Build history of the part. All positions in model axes, mm. A direction names the side the tool comes from. Coordinates: 2 decimals unless noted, no trailing zeros. Loops run counter-clockwise (first coordinate to the right, second up) from the corner with the lowest first, then second, coordinate; pieces in that order, holes last.
Item 1: Mould opens along Z. For faces 1 (the face through (12.524, 0.986, -39.192)), 2 (the face through (-27.62, 1.01, 53.6)), 3 (the face through (-13.3, 2, 15.6)) say: released by +Z, released by -Z, zero draft, split by the parting line, or undercut.
Item 2: Drill centre lines: line 1 along X through (y, z) = (0.85, 50); line 2 along Z through (x, y) = (2.5, 0.3); line 3 along Z through (x, y) = (10, 0.25). Where is each one in solid material? Low to high.
Item 3: Cut at A-A (x = -6). List the corners of the cut face in (y, z), and give its area (3 significant figures).
Item 4: Cut at C-C (z = 33). List the corners of the cut face in (x, y), and give its area (3 significant figures).
Item 5: Cut at D-D (y = 0.6). Count the separate pieces of the cut face and the enclosed holes in it, and give its area (3 significant figures).
Item 6: 3-axis set-ups, long thin cutter, end or side, ignore diameter. For faces 4 (the face through (29.05, 1, 6)), 5 (the face through (-10.781, -0.507, -8.774)), 6 (the face through (-12.5, 0.99, -15.54)): which of +Z, -Z, +X, -X, +Y, -Y reach the whole face in a straight line?
Item 7: Cut at B-B (z = -27.9). List the corners of the cut face in (x, y).
from build123d import *
from build123d.topology import SkipClean

# Parameters (mm, degrees)
SKETCH3_W           = 58.1
SKETCH3_H           = 99.8
SKETCH3_R           = 1.1
SKETCH3_R_2         = 0.95
SKETCH3_R_3         = 1.4
BOSS_EXTRUDE1_DEPTH = 2
FILLET1_R           = 5
FILLET2_R           = 3
FILLET3_R           = 10
BOSS_EXTRUDE2_START = 1
SKETCH4_R           = 1.6
SKETCH4_R_2         = 0.95
BOSS_EXTRUDE2_DEPTH = 1


with BuildPart() as part:
    # Sketch3 → Boss-Extrude1 (new body)
    with BuildSketch(Plane(origin=(0, 0, 0), x_dir=(1, 0, 0), z_dir=(0, 1, 0))):
        with Locations((0, -5.2)):
            Rectangle(SKETCH3_W, SKETCH3_H)
        with Locations(Location((24.05, -50.1, 0), (0, 0, 270))):
            Circle(SKETCH3_R, mode=Mode.SUBTRACT)
        with Locations(Location((-10.3, -10.3, 0), (0, 0, 270))):
            Circle(SKETCH3_R_2, mode=Mode.SUBTRACT)
        with Locations(Location((13.5, 39.7, 0), (0, 0, 270))):
            Circle(SKETCH3_R, mode=Mode.SUBTRACT)
        with Locations(Location((-13.5, 39.7, 0), (0, 0, 270))):
            Circle(SKETCH3_R, mode=Mode.SUBTRACT)
        with Locations(Location((-24.05, -50.1, 0), (0, 0, 270))):
            Circle(SKETCH3_R, mode=Mode.SUBTRACT)
        with Locations(Location((-24.5, 27.9, 0), (0, 0, 270))):
            Circle(SKETCH3_R_3, mode=Mode.SUBTRACT)
        with Locations(Location((24.5, 27.9, 0), (0, 0, 270))):
            Circle(SKETCH3_R_3, mode=Mode.SUBTRACT)
        with Locations(Location((10.3, 10.3, 0), (0, 0, 270))):
            Circle(SKETCH3_R_2, mode=Mode.SUBTRACT)
        with Locations(Location((10.3, -10.3, 0), (0, 0, 270))):
            Circle(SKETCH3_R_2, mode=Mode.SUBTRACT)
        with Locations(Location((-10.3, 10.3, 0), (0, 0, 270))):
            Circle(SKETCH3_R_2, mode=Mode.SUBTRACT)
        with Locations(Location((-24.5, -30.1, 0), (0, 0, 270))):
            Circle(SKETCH3_R_3, mode=Mode.SUBTRACT)
        with Locations(Location((24.5, -30.1, 0), (0, 0, 270))):
            Circle(SKETCH3_R_3, mode=Mode.SUBTRACT)
        with BuildLine():
            Line((19.05, -45.1), (19.05, -22.090559159))
            Line((19.05, -22.090559159), (8.77972042, -11.82027958))
            ThreePointArc((8.77972042, -11.82027958), (8.77972042, -8.77972042), (11.82027958, -8.77972042))
            Line((11.82027958, -8.77972042), (19.05, -16.009440841))
            Line((19.05, -16.009440841), (19.05, 16.009440841))
            Line((19.05, 16.009440841), (11.82027958, 8.77972042))
            ThreePointArc((11.82027958, 8.77972042), (8.77972042, 8.77972042), (8.77972042, 11.82027958))
            Line((8.77972042, 11.82027958), (19.05, 22.090559159))
            Line((19.05, 22.090559159), (19.05, 34.7))
            Line((19.05, 34.7), (-19.05, 34.7))
            Line((-19.05, 34.7), (-19.05, 22.090559159))
            Line((-19.05, 22.090559159), (-8.77972042, 11.82027958))
            ThreePointArc((-8.77972042, 11.82027958), (-8.77972042, 8.77972042), (-11.82027958, 8.77972042))
            Line((-11.82027958, 8.77972042), (-19.05, 16.009440841))
            Line((-19.05, 16.009440841), (-19.05, -16.009440841))
            Line((-19.05, -16.009440841), (-11.82027958, -8.77972042))
            ThreePointArc((-11.82027958, -8.77972042), (-8.77972042, -8.77972042), (-8.77972042, -11.82027958))
            Line((-8.77972042, -11.82027958), (-19.05, -22.090559159))
            Line((-19.05, -22.090559159), (-19.05, -45.1))
            Line((-19.05, -45.1), (19.05, -45.1))
        make_face(mode=Mode.SUBTRACT)
    extrude(amount=BOSS_EXTRUDE1_DEPTH)

    # Fillet1
    fillet1_edges = [part.edges().sort_by_distance(p)[0] for p in [
        (19.05, 1, -34.7),
        (-19.05, 1, -34.7),
        (-19.05, 1, 45.1),
        (19.05, 1, 45.1),
        (29.05, 1, -44.7),
        (29.05, 1, 55.1),
        (-29.05, 1, 55.1),
        (-29.05, 1, -44.7),
    ]]
    fillet(fillet1_edges, radius=FILLET1_R)

    # Fillet2
    fillet2_edges = [part.edges().sort_by_distance(p)[0] for p in [
        (-19.05, 1, -16.009440841),
        (-19.05, 1, 16.009440841),
        (19.05, 1, 16.009440841),
        (19.05, 1, -16.009440841),
    ]]
    fillet(fillet2_edges, radius=FILLET2_R)

    # Fillet3
    fillet3_edges = [part.edges().sort_by_distance(p)[0] for p in [
        (19.05, 1, -22.090559159),
        (-19.05, 1, -22.090559159),
        (-19.05, 1, 22.090559159),
        (19.05, 1, 22.090559159),
    ]]
    fillet(fillet3_edges, radius=FILLET3_R)

    # Sketch4 → Boss-Extrude2 (add)
    # profile 1 of 4: a face of its own
    with SkipClean():  # the faces are left unmerged after this step: merging them gives an invalid solid
        with BuildSketch(Plane.XZ.offset(BOSS_EXTRUDE2_START)):
            with Locations(Location((-10.3, 10.3, 0), (0, 0, 90))):
                Circle(SKETCH4_R)
            with Locations(Location((-10.3, 10.3, 0), (0, 0, 270))):
                Circle(SKETCH4_R_2, mode=Mode.SUBTRACT)
        # profile 2 of 4: a face of its own
        with BuildSketch(Plane.XZ.offset(BOSS_EXTRUDE2_START)):
            with Locations(Location((10.3, 10.3, 0), (0, 0, 90))):
                Circle(SKETCH4_R)
            with Locations(Location((10.3, 10.3, 0), (0, 0, 270))):
                Circle(SKETCH4_R_2, mode=Mode.SUBTRACT)
        # profile 3 of 4: a face of its own
        with BuildSketch(Plane.XZ.offset(BOSS_EXTRUDE2_START)):
            with Locations(Location((10.3, -10.3, 0), (0, 0, 90))):
                Circle(SKETCH4_R)
            with Locations(Location((10.3, -10.3, 0), (0, 0, 270))):
                Circle(SKETCH4_R_2, mode=Mode.SUBTRACT)
        # profile 4 of 4: a face of its own
        with BuildSketch(Plane.XZ.offset(BOSS_EXTRUDE2_START)):
            with Locations(Location((-10.3, -10.3, 0), (0, 0, 90))):
                Circle(SKETCH4_R)
            with Locations(Location((-10.3, -10.3, 0), (0, 0, 270))):
                Circle(SKETCH4_R_2, mode=Mode.SUBTRACT)
        extrude(amount=-BOSS_EXTRUDE2_DEPTH)


solid = part.part
Filled sheet:
1. face 1: undercut
1. face 2: released by +Z
1. face 3: zero draft
2. line 1: x = -29.05 to -25.15, -22.95 to 22.95, 25.15 to 29.05
2. line 2: z = -44.7 to -34.7, 45.1 to 55.1
2. line 3: z = -44.7 to -34.7, -13.04 to -11.2, -9.4 to -8.17, 8.17 to 9.4, 11.2 to 13.04, 45.1 to 55.1
3. outline: (0, -44.7) - (2, -44.7) - (2, -34.7) - (0, -34.7) - close; (0, 45.1) - (2, 45.1) - (2, 55.1) - (0, 55.1) - close
3. area: 40.0 mm2
4. outline: (-29.05, 0) - (-19.05, 0) - (-19.05, 2) - (-29.05, 2) - close; (19.05, 0) - (29.05, 0) - (29.05, 2) - (19.05, 2) - close
4. area: 40.0 mm2
5. separate pieces: 1
5. enclosed holes: 13
5. area: 3,000 mm2
6. face 4: +Z, -Z, +X, +Y, -Y
6. face 5: -Y
6. face 6: +Y, -Y
7. outline: (-29.05, 0) - (-25.9, 0) - (-25.9, 2) - (-29.05, 2) - close; (-23.1, 0) - (-19.05, 0) - (-19.05, 2) - (-23.1, 2) - close; (19.05, 0) - (23.1, 0) - (23.1, 2) - (19.05, 2) - close; (25.9, 0) - (29.05, 0) - (29.05, 2) - (25.9, 2) - close
